```python
from build123d import *

# Parameters (mm, degrees)
SKETCH_1_R          = 46
EXTRUDE_1_DEPTH     = 28.5
FILLET_1_R          = 8
SKETCH_2_R          = 1.5
CUT_EXTRUDE_1_DEPTH = 4
SKETCH_3_R          = 1.5
EXTRUDE_2_DEPTH     = 6
SKETCH_5_R          = 2
CUT_EXTRUDE_2_DEPTH = 4
CUT_EXTRUDE_3_DEPTH = 12
SKETCH_7_W          = 40
SKETCH_7_H          = 15


with BuildPart() as part:
    # 草图1 → 凸台-拉伸1 (new body)
    with BuildSketch(Plane.XY):
        with Locations(Location((0, 0, 0), (0, 0, 180))):
            Circle(SKETCH_1_R)
    extrude(amount=EXTRUDE_1_DEPTH)

    # 圆角1
    fillet_1_edges = [part.edges().sort_by_distance(p)[0] for p in [
        (46, 0, 0),
        (46, 0, 28.5),
    ]]
    fillet(fillet_1_edges, radius=FILLET_1_R)

    # 草图2 → 切除-拉伸1 (cut)
    with BuildSketch(Plane.XY.offset(28.5)):
        with Locations((0, -15.5)):
            Circle(SKETCH_2_R)
        with Locations((-15.5, 0)):
            Circle(SKETCH_2_R)
        with Locations((0, 15.5)):
            Circle(SKETCH_2_R)
        with Locations((15.5, 0)):
            Circle(SKETCH_2_R)
    extrude(amount=-CUT_EXTRUDE_1_DEPTH, mode=Mode.SUBTRACT)

    # 草图3 → 凸台-拉伸2 (add)
    with BuildSketch(Plane.XY.offset(28.5)):
        Circle(SKETCH_3_R)
    extrude(amount=EXTRUDE_2_DEPTH)

    # 草图5 → 切除-拉伸2 (cut)
    with BuildSketch(Plane(origin=(0, 0, 0), x_dir=(-1, 0, 0), z_dir=(0, 0, -1))):
        with Locations((-20, 0)):
            Circle(SKETCH_5_R)
        with Locations((0, 20)):
            Circle(SKETCH_5_R)
        with Locations((20, 0)):
            Circle(SKETCH_5_R)
        with Locations((0, -20)):
            Circle(SKETCH_5_R)
    extrude(amount=-CUT_EXTRUDE_2_DEPTH, mode=Mode.SUBTRACT)

    # 草图6 → 切除-拉伸3 (cut)
    with BuildSketch(Plane.XY.offset(28.5)):
        with BuildLine():
            Line((-1.935483871, -19.906127252), (-3.677419355, -37.821641779))
            ThreePointArc((-3.677419355, -37.821641779), (-19, -32.908965344), (-30.915792916, -22.095559471))
            Line((-30.915792916, -22.095559471), (-16.271469956, -11.629241827))
            ThreePointArc((-16.271469956, -11.629241827), (-10, -17.320508076), (-1.935483871, -19.906127252))
        make_face()
        with BuildLine():
            Line((1.935483871, -19.906127252), (3.677419355, -37.821641779))
            ThreePointArc((3.677419355, -37.821641779), (19, -32.908965344), (30.915792916, -22.095559471))
            Line((30.915792916, -22.095559471), (16.271469956, -11.629241827))
            ThreePointArc((16.271469956, -11.629241827), (10, -17.320508076), (1.935483871, -19.906127252))
        make_face()
        with BuildLine():
            Line((-18.206953827, -8.276885425), (-34.593212271, -15.726082308))
            ThreePointArc((-34.593212271, -15.726082308), (-38, 0), (-34.593212271, 15.726082308))
            Line((-34.593212271, 15.726082308), (-18.206953827, 8.276885425))
            ThreePointArc((-18.206953827, 8.276885425), (-19.999999876, 0), (-18.206953827, -8.276885425))
        make_face()
        with BuildLine():
            Line((-16.271469956, 11.629241827), (-30.915792916, 22.095559471))
            ThreePointArc((-30.915792916, 22.095559471), (-19, 32.908965344), (-3.677419355, 37.821641779))
            Line((-3.677419355, 37.821641779), (-1.935483871, 19.906127252))
            ThreePointArc((-1.935483871, 19.906127252), (-10, 17.320508076), (-16.271469956, 11.629241827))
        make_face()
        with BuildLine():
            Line((1.935483871, 19.906127252), (3.677419355, 37.821641779))
            ThreePointArc((3.677419355, 37.821641779), (19, 32.908965344), (30.915792916, 22.095559471))
            Line((30.915792916, 22.095559471), (16.271469956, 11.629241827))
            ThreePointArc((16.271469956, 11.629241827), (10, 17.320508076), (1.935483871, 19.906127252))
        make_face()
        with BuildLine():
            Line((18.206953827, 8.276885425), (34.593212271, 15.726082308))
            ThreePointArc((34.593212271, 15.726082308), (38, 0), (34.593212271, -15.726082308))
            Line((34.593212271, -15.726082308), (18.206953827, -8.276885425))
            ThreePointArc((18.206953827, -8.276885425), (20, 0), (18.206953827, 8.276885425))
        make_face()
    extrude(amount=-CUT_EXTRUDE_3_DEPTH, mode=Mode.SUBTRACT)

    # 草图7 → 切除-旋转1 (revolve, cut)
    with BuildSketch(Plane(origin=(0, 0, 0), x_dir=(1, 0, 0), z_dir=(0, 1, 0)), mode=Mode.PRIVATE) as cut_revolve_1_sk:
        with Locations((-20, -19)):
            Rectangle(SKETCH_7_W, SKETCH_7_H)
    revolve(cut_revolve_1_sk.sketch.rotate(Axis((0, 0, 28.5), (0, 0, -1)), 180), axis=Axis((0, 0, 28.5), (0, 0, -1)), mode=Mode.SUBTRACT)


solid = part.part
```
Part model, mm, in its own coordinate system. A direction names the side the tool comes from. Round coordinates to 2 decimals unless told otherwise and drop trailing zeros. Write each loop counter-clockwise with the first axis right and the second up, starting at its lowest first coordinate (ties: lowest second). Pieces come first, ordered by that corner, then holes. Notation, with made-up numbers: M 37,15 L 87,15 A27 ccw 87,39 Z; hole C 56.25,1 d7. An arc over 180 degrees is marked long. Answer as CSV lines item,"result". Start each with the question number.
1) Mould opens along Y. For faces 1 (the face through (18.803, 33.022, 27.514)), 2 (the face through (1, -1, 0)), 3 (the face through (5.99, -45.61, 14.16)) say: +Y half, -Y half, draft (parallel to the pull), parting line (faces both ways), or undercut.
2) Drill centre lines: L1, parallel to X at y = 24.5, z = 27.5; L2, parallel to Y at x = 0, z = 27.3; L3, parallel to Z at x = 31, y = 20.5. Where is each one in solid material? Low to high.
3) Band-saw the part on A-A (y = 0). Count the separate pieces of the cut face and the enclosed holes in it, then the cut area to 3 significant figures.
4) Drop flat-ended pins along their axis: pin 1 (12 mm diameter, centred on x = 15, y = -24, fed in from +Z); pin 2 (10 mm diameter, centred on x = 24, y = -23.5, fed in from +Z); pin 3 (4.5 mm diameter, centred on x = -20, y = 0, fed in from -Z); pin 4 (10 mm diameter, centred on y = -23, z = 22, fed in from +X). Give the stop position or say it passes through.
5) Band-saw the part on B-B (z = 9.5). List the corners of the cut face in (x, y), then the cut area to 3 significant figures.
6) Which spindle directions (+Z, -Z, +X, -X, +Y, -Y) get a long thin tool onto all of the face, cutting with end or side? Do faces 4 (the face through (0, 0, 34.5)), 5 (the face through (0, -18, 2)), 6 (the face through (-1, -1, 11.5)), 7 (the face through (14, 0, 28)). Say none if no direction does.
Worked out:
1,face 1,"undercut"
1,face 2,"draft"
1,face 3,"parting line"
2,L1,"-33.96 to -29.05, -2.38 to 2.38, 29.05 to 33.96"
2,L2,"-42.21 to -17, -14 to 14, 17 to 42.21"
2,L3,"0 to 11.5, 26.5 to 28.5"
3,separate pieces,"4"
3,enclosed holes,"0"
3,area,"1,270 mm²"
4,pin 1,"z = 11.5"
4,pin 2,"z = 28.5"
4,pin 3,"z = 0"
4,pin 4,"x = 42.27"
5,outline,"C 0,0 d92"
5,area,"6,650 mm²"
6,face 4,"+Z, +X, -X, +Y, -Y"
6,face 5,"-Z"
6,face 6,"none"
6,face 7,"+Z"
